from build123d import *

# Parameters (mm, degrees)
F1_DEPTH = 40
F3_DEPTH = 50
F5_DEPTH = 10
F7_DEPTH = 10
F8_R     = 15
F9_DEPTH = 10
F11_D    = 16


with BuildPart() as f1:
    # F0 (on Front) → F1 (new body)
    with BuildSketch(Plane.XZ):
        Polygon((35, 0), (-35, 0), (-35, -10), (-15, -10), (-15, -20), (15, -20), (15, -10), (35, -10), align=None)
    extrude(amount=F1_DEPTH)

    # F2 (on face) → F3 (join)
    with BuildSketch(Plane.XY):
        Polygon((35, 0), (-35, 0), (-35, -10), (25, -10), (25, -40), (35, -40), align=None)
    extrude(amount=F3_DEPTH)

    # F4 (on face) → F5 (cut, through all)
    with BuildSketch(Plane.XZ.offset(10)):
        Polygon((-15, 50), (-35, 50), (-35, 0), align=None)
    extrude(amount=-F5_DEPTH, mode=Mode.SUBTRACT)

    # F6 (on face) → F7 (cut, through all)
    with BuildSketch(Plane(origin=(25, 0, 0), x_dir=(0, -1, 0), z_dir=(-1, 0, 0))):
        Polygon((40, 50), (10, 50), (40, 0), align=None)
    extrude(amount=-F7_DEPTH, mode=Mode.SUBTRACT)

    # F8 (on face) → F9 (join)
    with BuildSketch(Plane.XZ.offset(10)):
        with Locations((0, 25)):
            Circle(F8_R)
    extrude(amount=F9_DEPTH)

    # F11 (through all)
    with Locations(Plane.XZ.offset(20)):
        with Locations((0, 25)):
            Hole(F11_D / 2)


solid = f1.part
Verification items for the finished model (mm, model axes). A direction names the side the tool comes from. Give positions to 0.01 mm unless a question says otherwise; leave off trailing zeros. Loops run counter-clockwise (first coordinate to the right, second up) from the corner with the lowest first, then second, coordinate; pieces in that order, holes last.
1) Sectioned sample at C-C, the plane y = -5.5. Enter the section's corners in (x, z), then the cut area to 3 significant figures.
2) Depth check by flat-ended pin: pin 1 Ø24 at (x, z) = (0.5, 18) entering from -Y; pin 2 Ø8 at (y, z) = (-25.5, -15.5) entering from +X; pin 3 Ø16 at (x, y) = (27.5, -26) entering from -Z; pin 4 Ø5 at (x, z) = (-23.5, 39.5) entering from -Y. Enter the tip coordinate at first touch or a pass-through.
3) Thickness scan on line 1 along Z through (x, y) = (0, -11); line 2 along Z through (x, y) = (-20.5, -35); line 3 along X through (y, z) = (-13, 32). Record the ranges inside material, lowest first.
4) Set-up check for faces 1 (the flat face through (1, -10, 8)), 2 (the flat face through (25, -21, 19)), 3 (the flat face through (15, -20, -15)), 4 (the flat face through (-25, -20, -10)), 5 (the flat face through (6, -20, 19)): record each of +Z, -Z, +X, -X, +Y, -Y from which the full face is reachable in a straight line by a thin tool's end or side.
5) Draft check along X on faces 6 (the cylindrical face through (1.041, -9.86, 32.932)), 7 (the flat face through (-35, -20, -5)), 8 (the flat face through (35, -16, 13)), 9 (the flat face through (0, -20, -20)). Enter one of: pulls with the +X half, pulls with the -X half, needs draft (parallel to the pull), parting line crosses it, or undercut.
6) Sectioned sample at B-B, the plane z = 25. Enter the section's corners in (x, y).
7) Sectioned sample at A-A, the plane y = -19. Enter the section's corners in (x, z).
8) Sectioned sample at D-D, the plane x = 0. Enter the section's corners in (y, z).
Answers:
1. outline: (-35, -10) - (-15, -10) - (-15, -20) - (15, -20) - (15, -10) - (35, -10) - (35, 50) - (-15, 50) - (-35, 0) - close; hole circle Ø16 at (0, 25)
1. area: 3,800 mm2
2. pin 1: stops at y = -20
2. pin 2: stops at x = 15
2. pin 3: stops at z = -10
2. pin 4: passes through
3. line 1: z = -20 to 0, 10 to 17, 33 to 40
3. line 2: z = -10 to 0
3. line 3: x = -13.27 to -3.87, 3.87 to 13.27, 25 to 35
4. face 1: -Y
4. face 2: +Z, -Y
4. face 3: -Z, +X, +Y, -Y
4. face 4: -Z, -X, +Y, -Y
4. face 5: +Z, -X, -Y
5. face 6: undercut
5. face 7: pulls with the -X half
5. face 8: pulls with the +X half
5. face 9: needs draft
6. outline: (-25, -10) - (-15, -10) - (-15, -20) - (-8, -20) - (-8, 0) - (-25, 0) - close; (8, -20) - (15, -20) - (15, -10) - (25, -10) - (25, -25) - (35, -25) - (35, 0) - (8, 0) - close
7. outline: (-35, -10) - (-15, -10) - (-15, -20) - (15, -20) - (15, -10) - (35, -10) - (35, 35) - (25, 35) - (25, 0) - (-35, 0) - close; circle Ø30 at (0, 25); hole circle Ø16 at (0, 25)
8. outline: (-40, -20) - (0, -20) - (0, 17) - (-20, 17) - (-20, 10) - (-10, 10) - (-10, 0) - (-40, 0) - close; (-20, 33) - (0, 33) - (0, 50) - (-10, 50) - (-10, 40) - (-20, 40) - close
